Answer from the drawing. Dimensions are ordinates in mm from the lowest x, y and z of the part. A direction names the side the tool comes from. Coordinates: 2 decimals unless noted, no trailing zeros. Write each loop counter-clockwise with the first axis right and the second up, starting at its lowest first coordinate (ties: lowest second). Pieces come first, ordered by that corner, then holes. Notation, with made-up numbers: (8.5, 46.5) -> (39.5, 46.5) arc R23 ccw to (39.5, 77.5) -> close; hole circle Ø7 at (76, 0). An arc over 180 degrees is marked (long way). One line per item, written item: value. Start each with the question number.
1. Find section C-C, the plane y = 3.25. Write down the section's boundary in (x, z).
2. Find section B-B, the plane z = 4.1. Write down the section's boundary in (x, y), and give its area (3 significant figures).
3. Consider line 1 along X through (y, z) = (2.5, 4.35); line 2 along Y through (x, z) = (2.5, 4.4); line 3 along Y through (x, z) = (11.08, 4.5). Determine where each line is inside the solid, lowest interval first.
4. Given P1, Ø3, axis at x = 11.08, y = 2.5, coming from the -Z side; P2, Ø8, axis at x = 11.5, y = 17.5, coming from the +Z side; P3, Ø0.9, axis at x = 3, z = 1.5, coming from the -Y side; P4, Ø2, axis at x = 7, z = 3.5, coming from the +Y side, each flat-ended and moving along its own axis, determine where each tip first touches the part or whether it passes through.
5. For a pull along Y with two mould halves and no side action, classify the marked faces 5, 6 and 7 as pulls with the +Y half, pulls with the -Y half, needs draft (parallel to the pull), parting line crosses it, or undercut.
6. Find section D-D, the plane z = 2.5. Write down the section's boundary in (x, y), and give its area (3 significant figures).
7. For the marked faces 1, 2, 3 and 4, determine the directions among +Z, -Z, +X, -X, +Y, -Y from which every point of the face is accessible in a straight line to the end or side of a thin tool.
8. Find section A-A, the plane x = 2.5. Write down the section's boundary in (y, z), and give its area (3 significant figures).
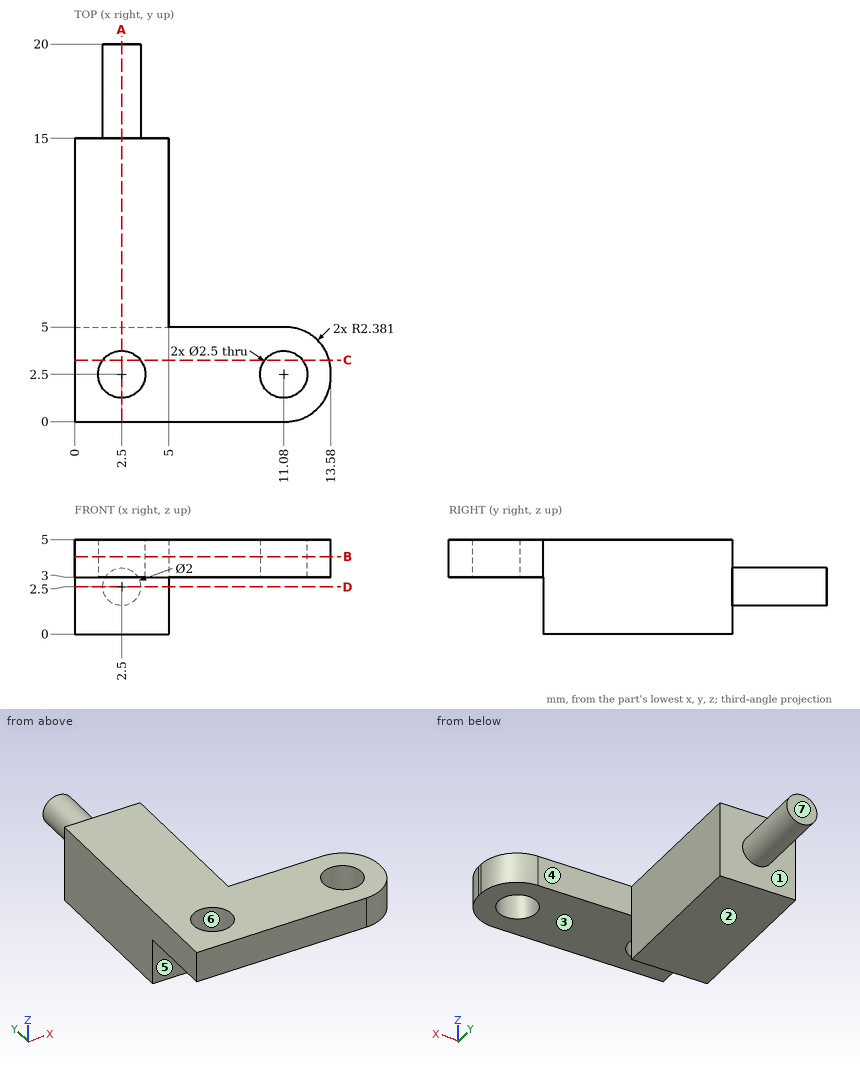
Answer block:
1. outline: (0, 3) -> (1.5, 3) -> (1.5, 5) -> (0, 5) -> close; (3.5, 3) -> (10.08, 3) -> (10.08, 5) -> (3.5, 5) -> close; (12.08, 3) -> (13.49, 3) -> (13.49, 5) -> (12.08, 5) -> close
2. outline: (0, 0) -> (11.2, 0) arc R2.38 ccw to (13.58, 2.38) -> (13.58, 2.62) arc R2.38 ccw to (11.2, 5) -> (5, 5) -> (5, 15) -> (0, 15) -> close; hole circle Ø2.5 at (2.5, 2.5); hole circle Ø2.5 at (11.08, 2.5)
2. area: 106 mm2
3. line 1: x = 0 to 1.25, 3.75 to 9.83, 12.33 to 13.58
3. line 2: y = 0 to 1.25, 3.75 to 15
3. line 3: y = 0 to 1.25, 3.75 to 5
4. P1: stops at z = 3
4. P2: passes through
4. P3: stops at y = 5
4. P4: stops at y = 5
5. face 5: pulls with the -Y half
5. face 6: undercut
5. face 7: pulls with the +Y half
6. outline: (0, 5) -> (5, 5) -> (5, 15) -> (3.5, 15) -> (3.5, 20) -> (1.5, 20) -> (1.5, 15) -> (0, 15) -> close
6. area: 60.0 mm2
7. face 1: +Y
7. face 2: -Z, +X, -X, +Y, -Y
7. face 3: -Z, +X, -X, -Y
7. face 4: +Z, -Z, +X, +Y
8. outline: (0, 3) -> (1.25, 3) -> (1.25, 5) -> (0, 5) -> close; (3.75, 3) -> (5, 3) -> (5, 0) -> (15, 0) -> (15, 1.5) -> (20, 1.5) -> (20, 3.5) -> (15, 3.5) -> (15, 5) -> (3.75, 5) -> close
8. area: 65.0 mm2
